Build history of the part. All positions in model axes, mm. Round coordinates to 2 decimals unless told otherwise and drop trailing zeros. One line per item, written item: value. Start each with the question number.
```python
from build123d import *

# Parameters (mm, degrees)
F0_R     = 1.2075
F0_R_2   = 1.2
F0_R_3   = 1.05
F0_R_4   = 0.4064
F0_R_5   = 0.2205357301
F0_R_6   = 0.08001
F1_DEPTH = 205
F2_R     = 1.05
F2_R_2   = 0.08001
F2_R_3   = 0.4064
F3_DEPTH = 1
F4_R     = 0.220535
F4_R_2   = 0.08001
F5_DEPTH = 1
F6_R     = 1.175
F6_R_2   = 1.05
F7_DEPTH = 0.5


with BuildPart() as f1:
    # F0 (on Front) → F1 (new body)
    with BuildSketch(Plane.XZ):
        with Locations((0, 0.2878)):
            Circle(F0_R)
        with Locations((0, 0.2878)):
            Circle(F0_R_2, mode=Mode.SUBTRACT)
        with Locations((0, 0.2878)):
            Circle(F0_R_2)
        with Locations((0, 0.2878)):
            Circle(F0_R_3, mode=Mode.SUBTRACT)
        with Locations((0, 0.2878)):
            Circle(F0_R_3)
        with BuildLine():
            add(Edge.make_bspline(
                [(0.2313024888, -0.5588), (0.2313024888, -0.3679270245), (-0.1156512444, -0.4633635122), (-0.4626049777, -0.5588), (-0.1156512444, -0.6542364878), (0.2313024888, -0.7496729755), (0.2313024888, -0.5588)],
                knots=[0, 0, 0, 2.0943951024, 2.0943951024, 4.1887902048, 4.1887902048, 6.2831853072, 6.2831853072, 6.2831853072], degree=2, weights=[1, 0.5, 1, 0.5, 1, 0.5, 1]))
        make_face(mode=Mode.SUBTRACT)
        Circle(F0_R_4, mode=Mode.SUBTRACT)
        with Locations((-0.5588, 0.4191)):
            Circle(F0_R_5, mode=Mode.SUBTRACT)
        with Locations((0, 0.8382)):
            Circle(F0_R_4, mode=Mode.SUBTRACT)
        with Locations((0.5588, 0.4191)):
            Circle(F0_R_5, mode=Mode.SUBTRACT)
        with Locations((-0.5588, 0.4191)):
            Circle(F0_R_5)
        with Locations((-0.65151, 0.318008)):
            Circle(F0_R_6, mode=Mode.SUBTRACT)
        with Locations((-0.65151, 0.51181)):
            Circle(F0_R_6, mode=Mode.SUBTRACT)
        with Locations((-0.46609, 0.4191)):
            Circle(F0_R_6, mode=Mode.SUBTRACT)
        with Locations((0.5588, 0.4191)):
            Circle(F0_R_5)
        with Locations((0.46609, 0.4191)):
            Circle(F0_R_6, mode=Mode.SUBTRACT)
        with Locations((0.65151, 0.318008)):
            Circle(F0_R_6, mode=Mode.SUBTRACT)
        with Locations((0.65151, 0.51181)):
            Circle(F0_R_6, mode=Mode.SUBTRACT)
        with BuildLine():
            add(Edge.make_bspline(
                [(0.2313024888, -0.5588), (0.2313024888, -0.3679270245), (-0.1156512444, -0.4633635122), (-0.4626049777, -0.5588), (-0.1156512444, -0.6542364878), (0.2313024888, -0.7496729755), (0.2313024888, -0.5588)],
                knots=[0, 0, 0, 2.0943951024, 2.0943951024, 4.1887902048, 4.1887902048, 6.2831853072, 6.2831853072, 6.2831853072], degree=2, weights=[1, 0.5, 1, 0.5, 1, 0.5, 1]))
        make_face()
        with Locations((-0.09271, -0.5588)):
            Circle(F0_R_6, mode=Mode.SUBTRACT)
        with Locations((0.09271, -0.5588)):
            Circle(F0_R_6, mode=Mode.SUBTRACT)
    extrude(amount=F1_DEPTH)

    # F2 (on face) → F3 (cut)
    with BuildSketch(Plane.XZ.offset(205)):
        with Locations((0, 0.2878)):
            Circle(F2_R)
        with Locations((-0.09271, -0.5588)):
            Circle(F2_R_2, mode=Mode.SUBTRACT)
        Circle(F2_R_3, mode=Mode.SUBTRACT)
        with Locations((0.09271, -0.5588)):
            Circle(F2_R_2, mode=Mode.SUBTRACT)
        with Locations((-0.65151, 0.318008)):
            Circle(F2_R_2, mode=Mode.SUBTRACT)
        with Locations((-0.65151, 0.51181)):
            Circle(F2_R_2, mode=Mode.SUBTRACT)
        with Locations((-0.46609, 0.4191)):
            Circle(F2_R_2, mode=Mode.SUBTRACT)
        with Locations((0, 0.8382)):
            Circle(F2_R_3, mode=Mode.SUBTRACT)
        with Locations((0.46609, 0.4191)):
            Circle(F2_R_2, mode=Mode.SUBTRACT)
        with Locations((0.65151, 0.318008)):
            Circle(F2_R_2, mode=Mode.SUBTRACT)
        with Locations((0.65151, 0.51181)):
            Circle(F2_R_2, mode=Mode.SUBTRACT)
    extrude(amount=-F3_DEPTH, mode=Mode.SUBTRACT)

    # F4 (on face) → F5 (cut)
    with BuildSketch(Plane.XZ.offset(204)):
        with Locations((-0.5588, 0.4191)):
            Circle(F4_R)
        with Locations((-0.65151, 0.318008)):
            Circle(F4_R_2, mode=Mode.SUBTRACT)
        with Locations((-0.65151, 0.51181)):
            Circle(F4_R_2, mode=Mode.SUBTRACT)
        with Locations((-0.46609, 0.4191)):
            Circle(F4_R_2, mode=Mode.SUBTRACT)
        with Locations((0.5588, 0.4191)):
            Circle(F4_R)
        with Locations((0.46609, 0.4191)):
            Circle(F4_R_2, mode=Mode.SUBTRACT)
        with Locations((0.65151, 0.318008)):
            Circle(F4_R_2, mode=Mode.SUBTRACT)
        with Locations((0.65151, 0.51181)):
            Circle(F4_R_2, mode=Mode.SUBTRACT)
        with BuildLine():
            add(Edge.make_bspline(
                [(0.2313, -0.5588), (0.2313, -0.3682744112), (-0.11565, -0.4635372056), (-0.4626, -0.5588), (-0.11565, -0.6540627944), (0.2313, -0.7493255888), (0.2313, -0.5588)],
                knots=[0, 0, 0, 2.0943951024, 2.0943951024, 4.1887902048, 4.1887902048, 6.2831853072, 6.2831853072, 6.2831853072], degree=2, weights=[1, 0.5, 1, 0.5, 1, 0.5, 1]))
        make_face()
        with Locations((-0.09271, -0.5588)):
            Circle(F4_R_2, mode=Mode.SUBTRACT)
        with BuildLine():
            ThreePointArc((0.0127, -0.5588), (0.09271, -0.47879), (0.17272, -0.5588))
            ThreePointArc((0.17272, -0.5588), (0.09271, -0.63881), (0.0127, -0.5588))
        make_face(mode=Mode.SUBTRACT)
    extrude(amount=-F5_DEPTH, mode=Mode.SUBTRACT)

    # F6 (on face) → F7 (cut)
    with BuildSketch(Plane.XZ.offset(205)):
        with Locations((0, 0.2878)):
            Circle(F6_R)
        with Locations((0, 0.2878)):
            Circle(F6_R_2, mode=Mode.SUBTRACT)
    extrude(amount=-F7_DEPTH, mode=Mode.SUBTRACT)


solid = f1.part
```
Item 1: Drill centre lines: line 1 (Z direction, x = -0.25, y = -111); line 2 (X direction, y = -170, z = 0.5); line 3 (X direction, y = -123, z = 0.2). Where is each one in solid material? Low to high.
Item 2: Drop a flat-ended pin along its axis: pin 1 (1 mm diameter, centred on y = -56.5, z = 0.5, fed in from -X). Give the stop position or say it passes through.
Item 3: Cut at A-A, the plane y = -156.5. Count the separate pieces of the cut face and the enclosed holes in it, plus the area to 3 significant figures.
Computed values:
1. line 1: z = -0.89 to -0.32, 0.32 to 0.52, 1.16 to 1.47
1. line 2: x = -1.19 to -0.73, -0.57 to -0.23, 0.23 to 0.57, 0.73 to 1.19
1. line 3: x = -1.2 to -0.35, 0.35 to 1.2
2. pin 1: stops at x = -1.21
3. separate pieces: 1
3. enclosed holes: 10
3. area: 3.38 mm2
